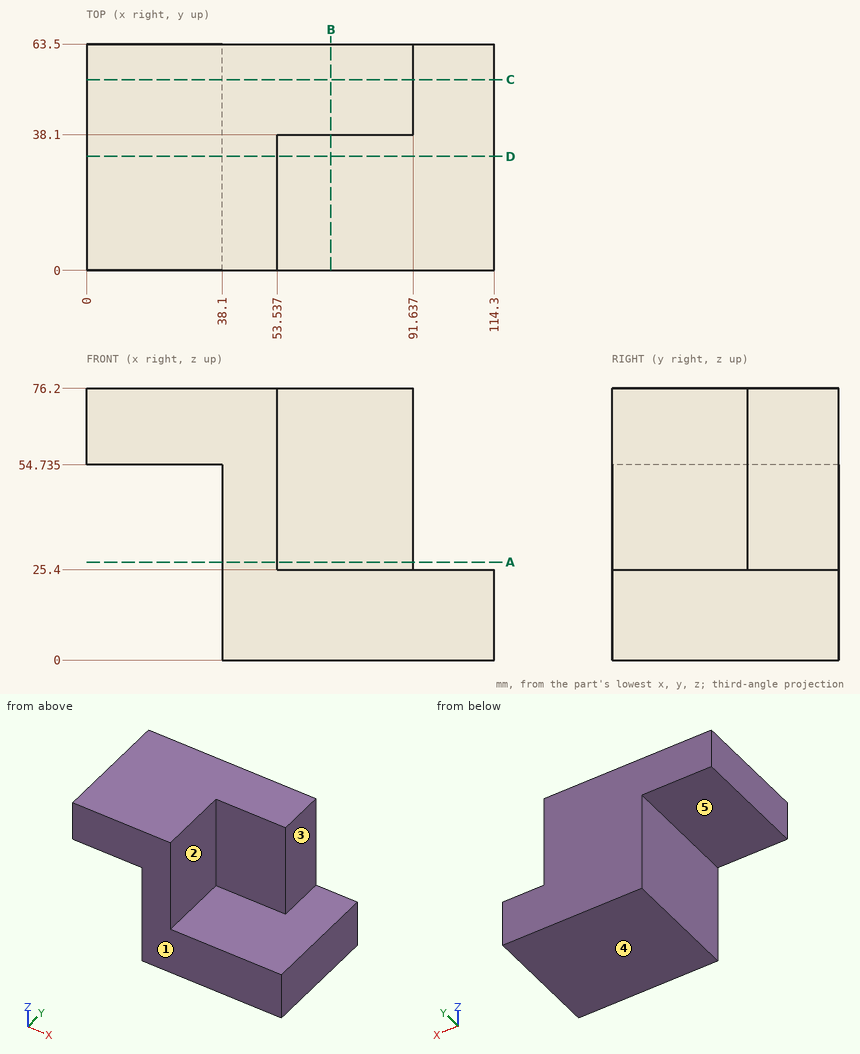
Input: dimensioned drawing with shaded views. Units: mm. Origin: part minimum x, y, z. A direction names the side the tool comes from. Coordinates: 2 decimals unless noted, no trailing zeros. Order: outer loops, then holes, each group sorted by start corner. A loop starts at its lowest first (then second) coordinate and runs counter-clockwise, first axis right, second up. Notation, with made-up numbers: (84, 31.5) -> (107, 31.5) arc R14 cw to (107, 49.5) -> close; hole circle Ø2 at (79, -4). An arc over 180 degrees is marked (long way). Use CSV: the item, a comma, the result in double quotes.
1) Section D-D on y = 32. Output: boundary loops of the cut face in (x, z) (1 decimal).
Findings:
outline,"(0, 54.7) -> (38.1, 54.7) -> (38.1, 0) -> (114.3, 0) -> (114.3, 25.4) -> (53.5, 25.4) -> (53.5, 76.2) -> (0, 76.2) -> close"
2) Access query for the marked faces 1, 2, 3, 4 and 5. Directions: +Z, -Z, +X, -X, +Y, -Y. A direction counts if a zero-diameter tool reaches every point of the face in a straight line with its end or side. Return the directions, or none.
Findings:
face 1,"+Z, -Z, +X, -X, -Y"
face 2,"+Z, +X, -Y"
face 3,"+Z, +X, +Y, -Y"
face 4,"-Z, +X, -X, +Y, -Y"
face 5,"-Z, -X, +Y, -Y"
3) Section A-A on z = 27.5. Output: boundary loops of the cut face in (x, y), then the cut area to 3 significant figures.
Findings:
outline,"(38.1, 0) -> (53.54, 0) -> (53.54, 38.1) -> (91.64, 38.1) -> (91.64, 63.5) -> (38.1, 63.5) -> close"
area,"1,950 mm^2"
4) Pin query (flat end, axial travel): pin 1 Ø11.5 at (y, z) = (11, 52) entering from +X; pin 2 Ø1.5 at (y, z) = (15.5, 11) entering from -X; pin 3 Ø2 at (x, z) = (81, 34) entering from -Y. Return the tip coordinate at first contact, or that it passes through.
Findings:
pin 1,"stops at x = 53.54"
pin 2,"stops at x = 38.1"
pin 3,"stops at y = 38.1"
5) Line query: line 1 (X direction, y = 4, z = 27.5); line 2 (X direction, y = 28, z = 70.5); line 3 (Y direction, x = 90.5, z = 61.5). Output: solid intervals per line, ascending.
Findings:
line 1,"x = 38.1 to 53.54"
line 2,"x = 0 to 53.54"
line 3,"y = 38.1 to 63.5"
6) Section B-B on x = 68.5. Output: boundary loops of the cut face in (y, z).
Findings:
outline,"(0, 0) -> (63.5, 0) -> (63.5, 76.2) -> (38.1, 76.2) -> (38.1, 25.4) -> (0, 25.4) -> close"
7) Section C-C on y = 53.5. Output: boundary loops of the cut face in (x, z) (1 decimal), then the cut area to 3 significant figures.
Findings:
outline,"(0, 54.7) -> (38.1, 54.7) -> (38.1, 0) -> (114.3, 0) -> (114.3, 25.4) -> (91.6, 25.4) -> (91.6, 76.2) -> (0, 76.2) -> close"
area,"5,470 mm^2"
